```python
from build123d import *

# Parameters (mm, degrees)
F0_W      = 76.2
F0_H      = 76.2
F1_DEPTH  = 12.7
F2_W      = 63.5
F2_H      = 63.5
F3_DEPTH  = 76.2
F6_T      = -2.54
F7_W      = 63.5
F7_H      = 63.5
F8_DEPTH  = 2.54
F9_R      = 25.4
F10_DEPTH = 25.4


# Not quite as in the source:
# - a feature of the source that left no trace in its solid (it failed there, or was rolled back) is left out


with BuildPart() as f1:
    # F0 (on Top) → F1 (new body)
    with BuildSketch(Plane.XY):
        Rectangle(F0_W, F0_H)
    extrude(amount=F1_DEPTH)

    # F2 (on face) → F3 (join)
    with BuildSketch(Plane.XY.offset(12.7)):
        Rectangle(F2_W, F2_H)
    extrude(amount=F3_DEPTH)

    # F6
    f6_openings = [f1.faces().sort_by_distance(p)[0] for p in [
        (0, 0, 88.9),
    ]]
    offset(amount=F6_T, openings=f6_openings, kind=Kind.INTERSECTION)

    # F7 (on face) → F8 (join)
    with BuildSketch(Plane.XY.offset(88.9)):
        Rectangle(F7_W, F7_H)
    extrude(amount=F8_DEPTH)

    # F9 (on face) → F10 (cut)
    with BuildSketch(Plane.XY.offset(91.44)):
        Circle(F9_R)
    extrude(amount=-F10_DEPTH, mode=Mode.SUBTRACT)


solid = f1.part
```
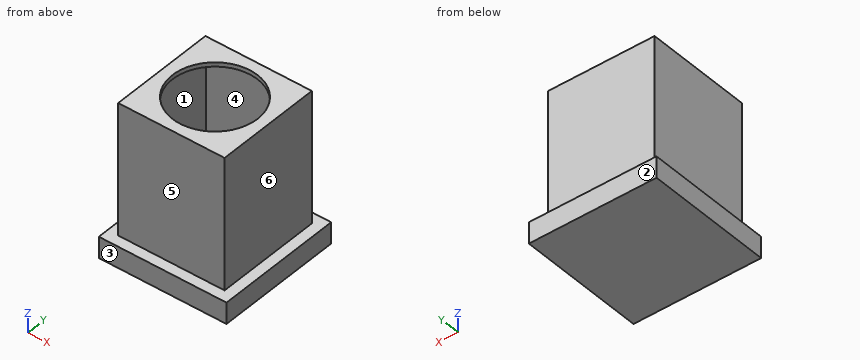
Check sheet for the modelled part. Datum: model origin and axes. Units: mm. Face numbers are marked on the shaded views. A direction names the side the tool comes from. Give positions to 0.01 mm unless a question says otherwise; leave off trailing zeros. Write each loop counter-clockwise with the first axis right and the second up, starting at its lowest first coordinate (ties: lowest second). Pieces come first, ordered by that corner, then holes. Notation, with made-up numbers: (-16.75, -31) - (-1.75, -31) arc R20 cw to (-1.75, 1) - close; hole circle Ø7 at (64.25, 80.25). An arc over 180 degrees is marked (long way). Answer as a JSON object with one key per item and string values. Group by question number.
1) Depth check by flat-ended pin: P1, Ø1.5, axis at x = 7.5, z = 13.5, coming from the -Y side; P2, Ø2, axis at x = -30, z = 31.5, coming from the +Y side; P3, Ø10, axis at y = -18, z = 20, coming from the -X side. Enter the tip coordinate at first touch or a pass-through.
2) Release check for a two-part mould opening along Y. For the marked faces 1, 2 and 3 record: pulls with the +Y half, pulls with the -Y half, needs draft (parallel to the pull), parting line crosses it, or undercut.
3) Sectioned sample at A-A (x = 0). Record the cut outline in (y, z).
4) Thickness scan on probe 1 along Y at (x, z) = (0, 90.05); probe 2 along X at (y, z) = (15.5, 5.5); probe 3 along X at (y, z) = (24, 70). Record the ranges inside material, lowest first. Write a range as from..to.
5) Access from +Z, -Z, +X, -X, +Y, -Y to the whole of each face (thin tool, end or side, straight path). Record for the marked faces 4, 5 and 6.
6) Sectioned sample at B-B (z = 68). Record the cut outline in (x, y), then the cut area to 3 significant figures.
Geometry results:
{
 "1": {"P1": "stops at y = -31.75", "P2": "stops at y = 31.75", "P3": "stops at x = -31.75"},
 "2": {"face 1": "undercut", "face 2": "pulls with the +Y half", "face 3": "pulls with the -Y half"},
 "3": {"outline": "(-38.1, 0) - (38.1, 0) - (38.1, 12.7) - (31.75, 12.7) - (31.75, 91.44) - (25.4, 91.44) - (25.4, 88.9) - (29.21, 88.9) - (29.21, 10.16) - (35.56, 10.16) - (35.56, 2.54) - (-35.56, 2.54) - (-35.56, 10.16) - (-29.21, 10.16) - (-29.21, 88.9) - (-25.4, 88.9) - (-25.4, 91.44) - (-31.75, 91.44) - (-31.75, 12.7) - (-38.1, 12.7) - close"},
 "4": {"probe 1": "y = -31.75..-25.4, 25.4..31.75", "probe 2": "x = -38.1..-35.56, 35.56..38.1", "probe 3": "x = -31.75..-29.21, 29.21..31.75"},
 "5": {"face 4": "none", "face 5": "+Z, +X, -X, -Y", "face 6": "+Z, +X, +Y, -Y"},
 "6": {"outline": "(-31.75, -31.75) - (31.75, -31.75) - (31.75, 31.75) - (-31.75, 31.75) - close; hole (-29.21, -29.21) - (29.21, -29.21) - (29.21, 29.21) - (-29.21, 29.21) - close", "area": "619 mm^2"}
}
